Could you check a few things on this drawing? It's one solid part, dimensions in mm from its lowest x, y, z. Give positions to 0.01 mm unless a question says otherwise; leave off trailing zeros. Loops run counter-clockwise (first coordinate to the right, second up) from the corner with the lowest first, then second, coordinate; pieces in that order, holes last.
Q1. Suppose I cut it at B-B (z = 47.5). List the corners of the cut face in (x, y) for me, and give its area (3 significant figures).
Q2. I need wall thicknesses on probe 1 along Z at (x, y) = (16.25, 2); probe 2 along X at (y, z) = (3, 56.5); probe 3 along Z at (x, y) = (15.5, 2.25). Which ranges of each line are inside material? Lowest first, please.
Q3. Suppose I cut it at A-A (x = 16.25). List the corners of the cut face in (y, z) for me.
Q4. I'm going to push a flat-ended pin straight in: P1, Ø2.5, axis at x = 6.25, z = 5.5, coming from the +Y side. Where does the tip first touch, or does it pass through?
Q5. Suppose I cut it at C-C (y = 4.75). Count the separate pieces of the cut face and the enclosed holes in it, and give its area (3 significant figures).
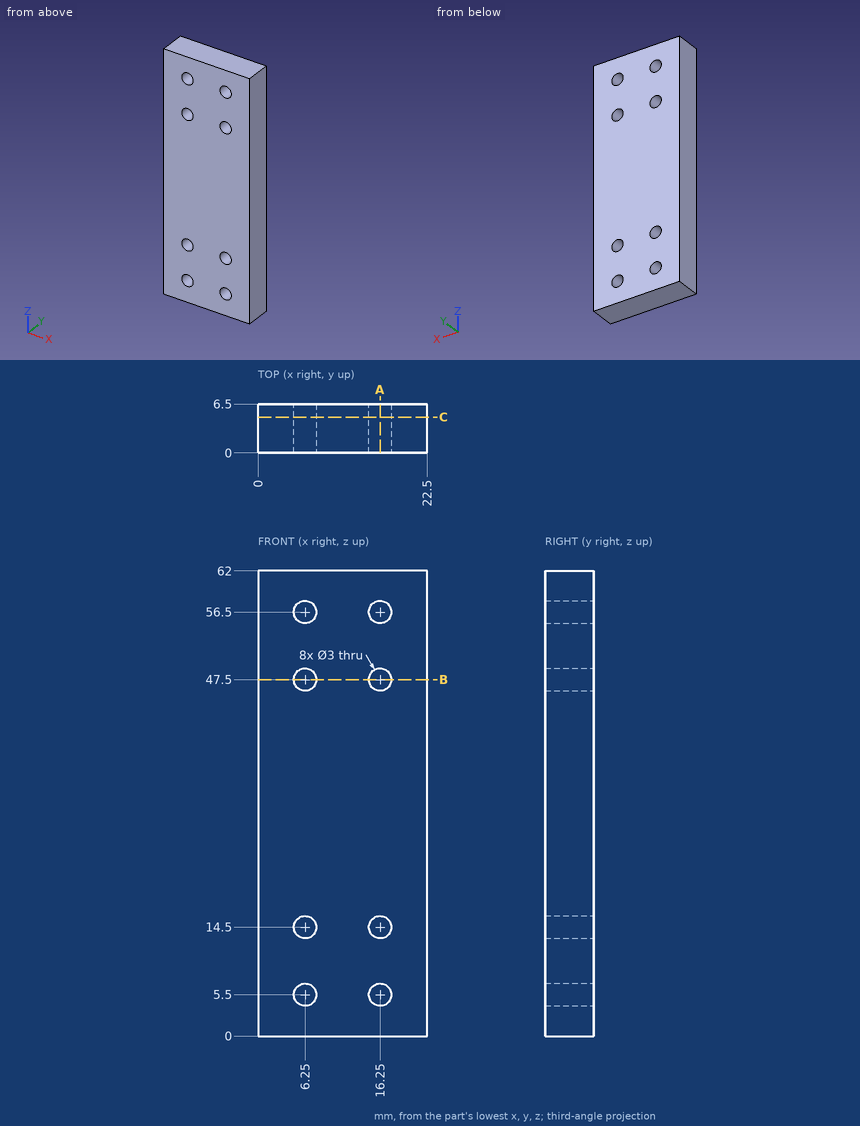
Solutions:
1. outline: (0, 0) - (4.75, 0) - (4.75, 6.5) - (0, 6.5) - close; (7.75, 0) - (14.75, 0) - (14.75, 6.5) - (7.75, 6.5) - close; (17.75, 0) - (22.5, 0) - (22.5, 6.5) - (17.75, 6.5) - close
1. area: 107 mm2
2. probe 1: z = 0 to 4, 7 to 13, 16 to 46, 49 to 55, 58 to 62
2. probe 2: x = 0 to 4.75, 7.75 to 14.75, 17.75 to 22.5
2. probe 3: z = 0 to 4.2, 6.8 to 13.2, 15.8 to 46.2, 48.8 to 55.2, 57.8 to 62
3. outline: (0, 0) - (6.5, 0) - (6.5, 4) - (0, 4) - close; (0, 7) - (6.5, 7) - (6.5, 13) - (0, 13) - close; (0, 16) - (6.5, 16) - (6.5, 46) - (0, 46) - close; (0, 49) - (6.5, 49) - (6.5, 55) - (0, 55) - close; (0, 58) - (6.5, 58) - (6.5, 62) - (0, 62) - close
4. P1: passes through
5. separate pieces: 1
5. enclosed holes: 8
5. area: 1,340 mm2
